```python
from build123d import *

# Parameters (mm, degrees)
SKETCH_W     = 35
SKETCH_H     = 16.7
SKETCH_R     = 1.6
PAD_DEPTH    = 1.5
SKETCH001_W  = 7.6
SKETCH001_H  = 10.5
PAD001_DEPTH = 7
SKETCH002_W  = 7.6
SKETCH002_H  = 10.5
PAD002_DEPTH = 3
PAD002_TAPER = 8
PAD003_DEPTH = 20


with BuildPart() as part:
    # Sketch → Pad (new body)
    with BuildSketch(Plane.XY):
        Rectangle(SKETCH_W, SKETCH_H)
        with Locations((-14.9, -5.75)):
            Circle(SKETCH_R, mode=Mode.SUBTRACT)
        with Locations((14.9, -5.75)):
            Circle(SKETCH_R, mode=Mode.SUBTRACT)
    extrude(amount=PAD_DEPTH)

    # Sketch001 (on Face8 of Pad) → Pad001 (join)
    with BuildSketch(Plane.XY.offset(1.5)):
        with Locations((-13.7, 3.1)):
            Rectangle(SKETCH001_W, SKETCH001_H)
        with Locations((13.7, 3.1)):
            Rectangle(SKETCH001_W, SKETCH001_H)
    extrude(amount=PAD001_DEPTH)

    # Sketch002 (on Face17 of Pad001) → Pad002 (join)
    with BuildSketch(Plane.XY.offset(8.5)):
        with Locations((-13.7, 3.1)):
            Rectangle(SKETCH002_W, SKETCH002_H)
        with Locations((13.7, 3.1)):
            Rectangle(SKETCH002_W, SKETCH002_H)
    extrude(amount=PAD002_DEPTH, taper=PAD002_TAPER)

    # Sketch003 (on Face5 of Pad002) → Pad003 (join)
    with BuildSketch(Plane.XY.offset(1.5)):
        Polygon((-7.5, 8.35), (-7.5, -1.85), (-5.6, -1.85), (-5.6, 6.45), (5.6, 6.45), (5.6, -1.85), (7.5, -1.85), (7.5, 8.35), align=None)
    extrude(amount=PAD003_DEPTH)


solid = part.part
```
Input: part model. Units: mm. Frame: model coordinates. A direction names the side the tool comes from. Coordinates: 2 decimals unless noted, no trailing zeros. Loops run counter-clockwise (first coordinate to the right, second up) from the corner with the lowest first, then second, coordinate; pieces in that order, holes last. Notation, with made-up numbers: (48, 52.5) - (89, 52.5) arc R13 ccw to (89, 64.5) - close; hole circle Ø6 at (-27.75, -40). An arc over 180 degrees is marked (long way). Answer in a Markdown table with one row per item.
(1) Cut plane C-C on x = 12.5. Output: boundary loops of the cut face in (y, z).
Model answer:
| item | result |
|---|---|
| outline | (-8.35, 0) - (8.35, 0) - (8.35, 8.5) - (7.93, 11.5) - (-1.73, 11.5) - (-2.15, 8.5) - (-2.15, 1.5) - (-8.35, 1.5) - close |
(2) Cut plane A-A on x = -14.9. Output: boundary loops of the cut face in (y, z).
Model answer:
| item | result |
|---|---|
| outline | (-8.35, 0) - (-7.35, 0) - (-7.35, 1.5) - (-8.35, 1.5) - close; (-4.15, 0) - (8.35, 0) - (8.35, 8.5) - (7.93, 11.5) - (-1.73, 11.5) - (-2.15, 8.5) - (-2.15, 1.5) - (-4.15, 1.5) - close |
(3) Set-up query: faces 1 (the face through (-14, 3, 11.5)), 2 (the face through (7, -1.85, 11)), 3 (the face through (14, 3, 11.5)), 4 (the face through (9.9, 3, 5)), 5 (the face through (-13.75, 8.14, 9.98)). Return all of +Z, -Z, +X, -X, +Y, -Y with unobstructed straight access to the full face (end or side cutting, diameter ignored); none if empty.
Model answer:
| item | result |
|---|---|
| face 1 | +Z, -X, +Y, -Y |
| face 2 | +Z, -Y |
| face 3 | +Z, +X, +Y, -Y |
| face 4 | +Z, +Y, -Y |
| face 5 | +Z, -X, +Y |
(4) Mould query, pull axis X, two halves, no side actions, for faces 6 (the face through (17.5, 2, 4)), 7 (the face through (-17.5, 2, 4)), 8 (the face through (0, 7, 21.5)), 9 (the face through (5.6, 2, 11)). Classes: pulls with the +X half, pulls with the -X half, needs draft (parallel to the pull), parting line crosses it, or undercut.
Model answer:
| item | result |
|---|---|
| face 6 | pulls with the +X half |
| face 7 | pulls with the -X half |
| face 8 | needs draft |
| face 9 | undercut |
(5) Cut plane D-D on z = 9.5. Output: boundary loops of the cut face in (x, y).
Model answer:
| item | result |
|---|---|
| outline | (-17.36, -2.01) - (-10.04, -2.01) - (-10.04, 8.21) - (-17.36, 8.21) - close; (-7.5, -1.85) - (-5.6, -1.85) - (-5.6, 6.45) - (5.6, 6.45) - (5.6, -1.85) - (7.5, -1.85) - (7.5, 8.35) - (-7.5, 8.35) - close; (10.04, -2.01) - (17.36, -2.01) - (17.36, 8.21) - (10.04, 8.21) - close |
(6) Material intervals for L1, parallel to X at y = 0.25, z = 4.75; L2, parallel to Y at x = 14.9, z = 0.5; L3, parallel to X at y = -0.5, z = 9.75, sorted ascending. Write a range as from..to.
Model answer:
| item | result |
|---|---|
| L1 | x = -17.5..-9.9, -7.5..-5.6, 5.6..7.5, 9.9..17.5 |
| L2 | y = -8.35..-7.35, -4.15..8.35 |
| L3 | x = -17.32..-10.08, -7.5..-5.6, 5.6..7.5, 10.08..17.32 |
(7) Cut plane B-B on z = 15.5. Output: boundary loops of the cut face in (x, y).
Model answer:
| item | result |
|---|---|
| outline | (-7.5, -1.85) - (-5.6, -1.85) - (-5.6, 6.45) - (5.6, 6.45) - (5.6, -1.85) - (7.5, -1.85) - (7.5, 8.35) - (-7.5, 8.35) - close |
(8) Pin query (flat end, axial travel): P1, Ø5, axis at x = 0.5, y = -2.5, coming from the +Z side; P2, Ø4, axis at y = 1, z = 15, coming from the +X side; P3, Ø5.5, axis at x = 14, y = 5.5, coming from the +Z side. Return the tip coordinate at first contact, or that it passes through.
Model answer:
| item | result |
|---|---|
| P1 | stops at z = 1.5 |
| P2 | stops at x = 7.5 |
| P3 | stops at z = 11.5 |
